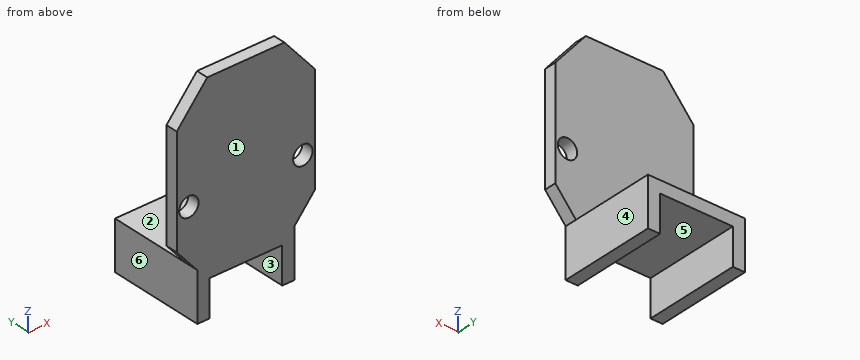
```python
from build123d import *
from OCP.BRepFilletAPI import BRepFilletAPI_MakeChamfer

# Parameters (mm, degrees)
SKETCH1_W           = 40
SKETCH1_H           = 40
BOSS_EXTRUDE1_DEPTH = 20
SKETCH2_W           = 30
SKETCH2_H           = 40
CUT_EXTRUDE1_DEPTH  = 15
SKETCH3_W           = 57
SKETCH3_H           = 5
BOSS_EXTRUDE2_DEPTH = 70
DRAFT1_ANGLE        = 50
DRAFT2_ANGLE        = 50
CHAMFER1_SIZE       = 15
CHAMFER1_SIZE2      = 12.586494468
SKETCH6_R           = 4
CUT_EXTRUDE3_DEPTH  = 109.061325182


with BuildPart() as part:
    # Sketch1 → Boss-Extrude1 (new body)
    with BuildSketch(Plane.XY):
        with Locations((20, 20)):
            Rectangle(SKETCH1_W, SKETCH1_H)
    extrude(amount=BOSS_EXTRUDE1_DEPTH)

    # Sketch2 → Cut-Extrude1 (cut)
    with BuildSketch(Plane(origin=(0, 0, 0), x_dir=(-1, 0, 0), z_dir=(0, 0, -1))):
        with Locations((-20, 20)):
            Rectangle(SKETCH2_W, SKETCH2_H)
    extrude(amount=-CUT_EXTRUDE1_DEPTH, mode=Mode.SUBTRACT)

    # Sketch3 → Boss-Extrude2 (add)
    with BuildSketch(Plane.XY.offset(20)):
        with Locations((20, 2.5)):
            Rectangle(SKETCH3_W, SKETCH3_H)
    extrude(amount=BOSS_EXTRUDE2_DEPTH)

    # Draft1
    draft1_faces = [part.faces().sort_by_distance(p)[0] for p in [
        (-4.25, 2.5, 20),
    ]]
    draft(draft1_faces, Plane(origin=(0, 0, 20), x_dir=(0, 0, -1), z_dir=(-1, 0, 0)), DRAFT1_ANGLE)

    # Draft2
    draft2_faces = [part.faces().sort_by_distance(p)[0] for p in [
        (44.25, 2.5, 20),
    ]]
    draft(draft2_faces, Plane(origin=(40, 40, 20), x_dir=(0, 1, 0), z_dir=(1, 0, 0)), DRAFT2_ANGLE)

    # Chamfer1: one chamfer whose edges measure the first distance from different faces: ONE call of the kernel's chamfer builder (chamfer() names one face for all edges)
    chamfer1_edges_1 = [part.edges().sort_by_distance(p)[0] for p in [
        (-8.5, 2.5, 90),
    ]]
    chamfer1_side_1 = [part.faces().sort_by_distance(p)[0] for p in [
        (-8.5, 2.5, 60.064952769),
    ]]
    chamfer1_edges_2 = [part.edges().sort_by_distance(p)[0] for p in [
        (48.5, 2.5, 90),
    ]]
    chamfer1_side_2 = [part.faces().sort_by_distance(p)[0] for p in [
        (48.5, 2.5, 60.064952769),
    ]]
    chamfer1 = BRepFilletAPI_MakeChamfer(part.part.solid().wrapped)
    for e in chamfer1_edges_1:
        chamfer1.Add(CHAMFER1_SIZE, CHAMFER1_SIZE2, e.wrapped, chamfer1_side_1[0].wrapped)  # the first distance lies on this face
    for e in chamfer1_edges_2:
        chamfer1.Add(CHAMFER1_SIZE, CHAMFER1_SIZE2, e.wrapped, chamfer1_side_2[0].wrapped)  # the first distance lies on this face
    add(Compound.cast(chamfer1.Shape()), mode=Mode.REPLACE)

    # Sketch6 → Cut-Extrude3 (cut, through all)
    with BuildSketch(Plane(origin=(0, 5, 0), x_dir=(1, 0, 0), z_dir=(0, 1, 0))):
        with Locations(Location((-3.5, -45, 0), (0, 0, 270))):
            Circle(SKETCH6_R)
        with Locations(Location((43.5, -45, 0), (0, 0, 90))):
            Circle(SKETCH6_R)
    extrude(amount=-CUT_EXTRUDE3_DEPTH, mode=Mode.SUBTRACT)


solid = part.part
```
The model under review builds one solid part; all positions refer to its coordinate system, in mm. Face numbers are marked on the shaded views. A direction names the side the tool comes from. Give positions to 0.01 mm unless a question says otherwise; leave off trailing zeros. Write each loop counter-clockwise with the first axis right and the second up, starting at its lowest first coordinate (ties: lowest second). Pieces come first, ordered by that corner, then holes. Notation, with made-up numbers: M 17.5,12 L 54.5,12 A17 cw 54.5,31 Z; hole C -29.5,-34 d10. An arc over 180 degrees is marked long. Write each question's results on one line, items separated by ' | '. Start each with the question number.
1. For the marked faces 1, 2 and 3, list the 3-axis set-ups (+Z, -Z, +X, -X, +Y, -Y) from which the entire face can be reached by the end or side of a thin tool; tool diameter is ignored.
2. We need section C-C (y = 28.5). Write out the cut boundary in (x, z).
3. Mouldability with a two-part tool opening along X and no side actions: class the marked faces 4, 5 and 6 as released by +X, released by -X, zero draft, split by the parting line, or undercut.
4. We need section A-A (z = 45). Write out the cut boundary in (x, y), and give its area (3 significant figures).
5. We need section B-B (x = -3.5). Write out the cut boundary in (y, z), and give its area (3 significant figures).
6. For probe 1 along X at (y, z) = (3, 45); probe 2 along Z at (x, y) = (-3, 3); probe 3 along Y at (x, z) = (26, 72), list the stretches that pass through material, from the lowest coordinate up. Write a range as [from, to].
7. We need section D-D (x = 23). Write out the cut boundary in (y, z).
8. Insertion check: pin 1 Ø1.5 at (x, y) = (30.5, 11) entering from +Z; pin 2 Ø9 at (x, z) = (-3.5, 45) entering from -Y; pin 3 Ø4.5 at (y, z) = (11.5, 7) entering from +X; pin 4 Ø6.5 at (x, z) = (43.5, 45) entering from +Y. Each pin has a flat end and moves straight along its axis. Give the tip position at first contact, or say it passes through.
Results found:
1) face 1: +Z, -Z, +X, -X, -Y | face 2: +Z, +X, -X, +Y | face 3: -Z, +Y, -Y
2) outline: M 0,0 L 5,0 L 5,15 L 35,15 L 35,0 L 40,0 L 40,20 L 0,20 Z
3) face 4: released by +X | face 5: undercut | face 6: released by -X
4) outline: M -8.5,0 L -7.5,0 L -7.5,5 L -8.5,5 Z; M 0.5,0 L 39.5,0 L 39.5,5 L 0.5,5 Z; M 47.5,0 L 48.5,0 L 48.5,5 L 47.5,5 Z | area: 205 mm^2
5) outline: M 0,24.17 L 5,24.17 L 5,41 L 0,41 Z; M 0,49 L 5,49 L 5,80.96 L 0,80.96 Z | area: 244 mm^2
6) probe 1: x = [-8.5, -7.5], [0.5, 39.5], [47.5, 48.5] | probe 2: z = [23.58, 41.03], [48.97, 81.55] | probe 3: y = [0, 5]
7) outline: M 0,15 L 40,15 L 40,20 L 5,20 L 5,90 L 0,90 Z
8) pin 1: stops at z = 20 | pin 2: stops at y = 0 | pin 3: stops at x = 40 | pin 4: passes through
